The listing builds one solid part. Answer for the finished solid, in the listing's coordinates (mm). A direction names the side the tool comes from. Round coordinates to 2 decimals unless told otherwise and drop trailing zeros. Order: outer loops, then holes, each group sorted by start corner. A loop starts at its lowest first (then second) coordinate and runs counter-clockwise, first axis right, second up. Notation, with made-up numbers: (19.25, -38) - (38.25, -38) arc R13 cw to (38.25, -32) - close; hole circle Ø9 at (32.25, 57.25). An arc over 180 degrees is marked (long way). Write item = value, one per line.
from build123d import *

# Parameters (mm, degrees)
SKETCH1_R           = 1.5
BOSS_EXTRUDE1_DEPTH = 3


with BuildPart() as part:
    # Sketch1 → Boss-Extrude1 (new body)
    with BuildSketch(Plane(origin=(0, 0, 0), x_dir=(1, 0, 0), z_dir=(0, 1, 0))):
        with BuildLine():
            Line((28, 5), (13.610657589, 5))
            ThreePointArc((13.610657589, 5), (-14.5, 0), (13.610657589, -5))
            Line((13.610657589, -5), (28, -5))
            ThreePointArc((28, -5), (33, 0), (28, 5))
        make_face()
        with Locations((28, 0)):
            Circle(SKETCH1_R, mode=Mode.SUBTRACT)
        Circle(SKETCH1_R, mode=Mode.SUBTRACT)
        with Locations((7, 0)):
            Circle(SKETCH1_R, mode=Mode.SUBTRACT)
        with Locations((-7, 0)):
            Circle(SKETCH1_R, mode=Mode.SUBTRACT)
    extrude(amount=BOSS_EXTRUDE1_DEPTH)


solid = part.part
Q1. Section D-D on x = 7 is taken. Determine the outline of the cut face in (y, z).
Model answer:
outline = (0, -12.7) - (3, -12.7) - (3, -1.5) - (0, -1.5) - close; (0, 1.5) - (3, 1.5) - (3, 12.7) - (0, 12.7) - close
Q2. Section B-B on z = 0 is taken. Determine the outline of the cut face in (x, y).
Model answer:
outline = (-14.5, 0) - (-8.5, 0) - (-8.5, 3) - (-14.5, 3) - close; (-5.5, 0) - (-1.5, 0) - (-1.5, 3) - (-5.5, 3) - close; (1.5, 0) - (5.5, 0) - (5.5, 3) - (1.5, 3) - close; (8.5, 0) - (26.5, 0) - (26.5, 3) - (8.5, 3) - close; (29.5, 0) - (33, 0) - (33, 3) - (29.5, 3) - close
Q3. Flat-ended cylindrical pins translate along their axes: P1, Ø1.5, axis at x = -9, y = 1, coming from the +Z side; P2, Ø1.5, axis at x = 27, y = 2.5, coming from the -Z side. Find the tip coordinate at first contact, or state that the pin passes through.
Model answer:
P1 = 11.92
P2 = -5
Q4. Determine the mould class of faces 3 (the face through (5.5, 1.48, -0.07)), 4 (the face through (-8.5, 1.48, -0.07)), 5 (the face through (33, 1, 0)), 6 (the face through (21, 1, -5)) for opening direction Z: released by +Z, released by -Z, zero draft, split by the parting line, or undercut.
Model answer:
face_3 = undercut
face_4 = undercut
face_5 = split by the parting line
face_6 = released by -Z
Q5. For faces 1 (the face through (-14.49, 1.48, -0.57)), 2 (the face through (21, 1, 5)), determine the directions among +Z, -Z, +X, -X, +Y, -Y from which every point of the face is accessible in a straight line to the end or side of a thin tool.
Model answer:
face_1 = +Y, -Y
face_2 = +Z, +X, +Y, -Y
Q6. Section A-A on y = 1 is taken. Determine the outline of the cut face in (x, z).
Model answer:
outline = (13.61, -5) - (28, -5) arc R5 ccw to (28, 5) - (13.61, 5) arc R14.5 ccw (long way) to start; hole circle Ø3 at (-7, 0); hole circle Ø3 at (0, 0); hole circle Ø3 at (7, 0); hole circle Ø3 at (28, 0)
Q7. Section C-C on x = 0 is taken. Determine the outline of the cut face in (y, z).
Model answer:
outline = (0, -14.5) - (3, -14.5) - (3, -1.5) - (0, -1.5) - close; (0, 1.5) - (3, 1.5) - (3, 14.5) - (0, 14.5) - close
Q8. Find the intervals of material crossed by line 1 (X direction, y = 1.25, z = 0); line 2 (Z direction, x = 0, y = 1.4); line 3 (X direction, y = 0.55, z = 0.5), in increasing order. Write a range as from..to.
Model answer:
line_1 = -14.5..-8.5, -5.5..-1.5, 1.5..5.5, 8.5..26.5, 29.5..33
line_2 = -14.5..-1.5, 1.5..14.5
line_3 = -14.49..-8.41, -5.59..-1.41, 1.41..5.59, 8.41..26.59, 29.41..32.97
